Part model, mm, in its own coordinate system. Face numbers are marked on the shaded views. A direction names the side the tool comes from. Coordinates: 2 decimals unless noted, no trailing zeros. Order: outer loops, then holes, each group sorted by start corner. A loop starts at its lowest first (then second) coordinate and runs counter-clockwise, first axis right, second up.
Autodesk Inventor part; units mm, degrees
ref_plane "YZ Plane" through (0, 0, 0) normal (1, 0, 0) x (0, 1, 0)
ref_plane "XZ Plane" through (0, 0, 0) normal (0, 1, 0) x (-1, 0, 0)
ref_plane "XY Plane" through (0, 0, 0) normal (0, 0, 1) x (1, 0, 0)
sketch "Sketch1" plane through (0, 0, 0) normal (0, 0, 1) x (1, 0, 0)
  line L0 (0, 0) -> (17.9, 0)
  line L1 (17.9, 0) -> (17.9, 14.7)
  line L2 (17.9, 14.7) -> (0, 14.7)
  line L3 (0, 14.7) -> (0, 0)
  dimension "d0" = 17.9
  dimension "d1" = 14.7
extrude "Extrusion1" add sketch "Sketch1" along normal blind 2
sketch "Sketch2" plane through (0, 0, 2) normal (0, 0, 1) x (1, 0, 0)
  line L0 (1.95, 0.5) -> (15.95, 0.5)
  line L1 (15.95, 0.5) -> (15.95, 5)
  line L2 (15.95, 5) -> (1.95, 5)
  line L3 (1.95, 5) -> (1.95, 0.5)
  line L4 (0, 0) -> (17.9, 0)
  line L5 (17.9, 0) -> (17.9, 14.7)
  line L6 (0, 14.7) -> (0, 0)
  line L7 (1.95, 9.7) -> (15.95, 9.7)
  line L8 (15.95, 9.7) -> (15.95, 14.2)
  line L9 (15.95, 14.2) -> (1.95, 14.2)
  line L10 (1.95, 14.2) -> (1.95, 9.7)
  line L11 (17.9, 14.7) -> (0, 14.7)
  dimension "d6" = 0.5
  dimension "d7" = 4.5
  dimension "d8" = 14
  dimension "d9" = 1.95
  dimension "d10" = 1.95
  dimension "d11" = 4.5
  dimension "d12" = 14
  dimension "d13" = 0.5
  dimension "d14" = 1.95
  dimension "d15" = 1.95
extrude "Extrusion2" add sketch "Sketch2" along normal blind 7.5 contours L3 L2 L1 L0 | L10 L9 L8 L7
properties part number "HDMI_Jumper"
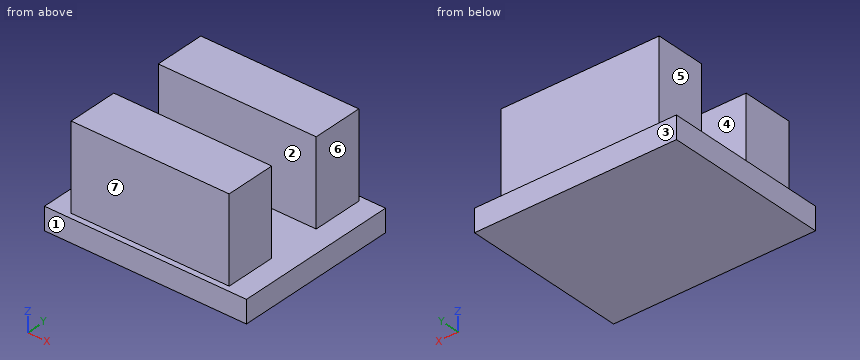
(1) Slice it at B-B, the plane x = 2.25. Give the cut face in (y, z).
(2) Probe line 1 (Y direction, x = 3.75, z = 4); line 2 (X direction, y = 3, z = 4); line 3 (Z direction, x = 2.75, y = 5.5). List the from-to ranges inside material, lowest first.
(3) Drop flat-ended pins along their axis: pin 1 (1.5 mm diameter, centred on y = 13, z = 4, fed in from -X); pin 2 (4 mm diameter, centred on x = 6, z = 7.5, fed in from +Y); pin 3 (3.5 mm diameter, centred on y = 11, z = 4.5, fed in from +X); pin 4 (3 mm diameter, centred on x = 3, y = 5, fed in from -Z). Give the stop position or say it passes through.
(4) Tool access for the marked faces 4, 5, 6 and 7: list every direction of +Z, -Z, +X, -X, +Y, -Y with a clear straight run to the whole face (end or side of a thin tool).
(5) Pull direction Y, two halves, no side cores. Call the marked faces 1, 2 and 3: +Y half, -Y half, draft (parallel to the pull), parting line (faces both ways), or undercut.
(6) Slice it at D-D, the plane y = 7. Give the cut face in (x, z).
(7) Slice it at C-C, the plane y = 3. Give the cut face in (x, z), then the cut area to 3 significant figures.
(8) Slice it at A-A, the plane z = 7.75. Give the cut face in (x, y).
Here are the results:
1. outline: (0, 0) - (14.7, 0) - (14.7, 2) - (14.2, 2) - (14.2, 9.5) - (9.7, 9.5) - (9.7, 2) - (5, 2) - (5, 9.5) - (0.5, 9.5) - (0.5, 2) - (0, 2) - close
2. line 1: y = 0.5 to 5, 9.7 to 14.2
2. line 2: x = 1.95 to 15.95
2. line 3: z = 0 to 2
3. pin 1: stops at x = 1.95
3. pin 2: stops at y = 14.2
3. pin 3: stops at x = 15.95
3. pin 4: stops at z = 0
4. face 4: +Z, +X, -X
4. face 5: +Z, -X, +Y, -Y
4. face 6: +Z, +X, +Y, -Y
4. face 7: +Z, +X, -X, -Y
5. face 1: -Y half
5. face 2: undercut
5. face 3: +Y half
6. outline: (0, 0) - (17.9, 0) - (17.9, 2) - (0, 2) - close
7. outline: (0, 0) - (17.9, 0) - (17.9, 2) - (15.95, 2) - (15.95, 9.5) - (1.95, 9.5) - (1.95, 2) - (0, 2) - close
7. area: 141 mm2
8. outline: (1.95, 0.5) - (15.95, 0.5) - (15.95, 5) - (1.95, 5) - close; (1.95, 9.7) - (15.95, 9.7) - (15.95, 14.2) - (1.95, 14.2) - close
